The drawing under review shows one solid part. Ordinate dimensions are in mm from its lowest x, y, z. A direction names the side the tool comes from. Round coordinates to 2 decimals unless told otherwise and drop trailing zeros. Loops run counter-clockwise (first coordinate to the right, second up) from the corner with the lowest first, then second, coordinate; pieces in that order, holes last. Notation, with made-up numbers: M 37.25,6.25 L 46.25,6.25 A29 cw 46.25,34.25 Z; hole C 55.25,-30.5 d9. An arc over 180 degrees is marked long. Use a Markdown table: item, result.
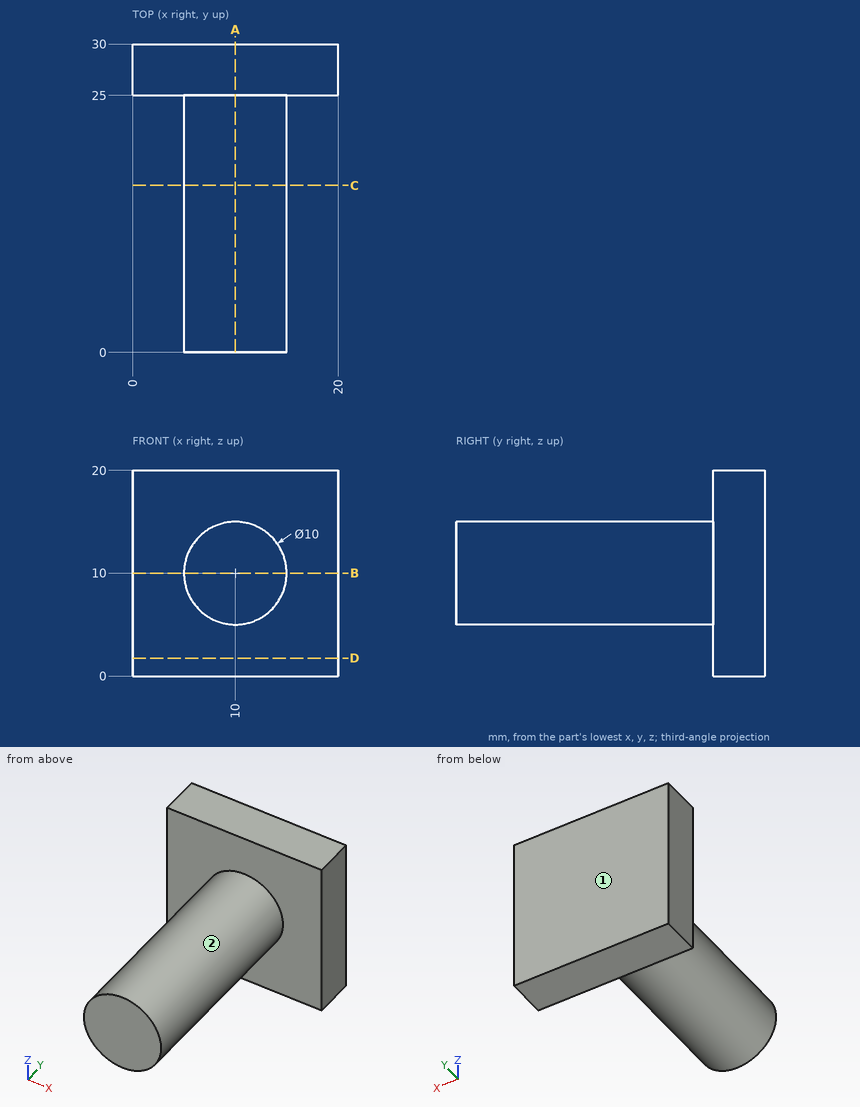
1. Take a section at D-D on z = 1.75. Give the boundary of the cut face in (x, y).
Check values:
| item | result |
|---|---|
| outline | M 0,25 L 20,25 L 20,30 L 0,30 Z |
2. Take a section at B-B on z = 10. Give the boundary of the cut face in (x, y), and give its area (3 significant figures).
Check values:
| item | result |
|---|---|
| outline | M 0,25 L 5,25 L 5,0 L 15,0 L 15,25 L 20,25 L 20,30 L 0,30 Z |
| area | 350 mm² |
3. Wall thickness on line 1 along Y through (x, z) = (15.5, 4.5); line 2 along Z through (x, y) = (7.5, 20); line 3 along X through (y, z) = (7.5, 9.25): over which ranges is each line inside the solid? List them lowest first. Write a range as from..to.
Check values:
| item | result |
|---|---|
| line 1 | y = 25..30 |
| line 2 | z = 5.67..14.33 |
| line 3 | x = 5.06..14.94 |
4. Take a section at A-A on x = 10. Give the boundary of the cut face in (y, z), and give its area (3 significant figures).
Check values:
| item | result |
|---|---|
| outline | M 0,5 L 25,5 L 25,0 L 30,0 L 30,20 L 25,20 L 25,15 L 0,15 Z |
| area | 350 mm² |
5. Take a section at C-C on y = 16.25. Give the boundary of the cut face in (x, z), and give its area (3 significant figures).
Check values:
| item | result |
|---|---|
| outline | C 10,10 d10 |
| area | 78.5 mm² |
6. Machinability: for the marked faces 1 and 2, which of the approach directions +Z, -Z, +X, -X, +Y, -Y give a long, thin tool a straight path to every point of the face, cutting with its end or side? Answer none if there is none.
Check values:
| item | result |
|---|---|
| face 1 | +Z, -Z, +X, -X, +Y |
| face 2 | -Y |
7. Insertion check: pin 1 (8 mm diameter, centred on x = 4.5, y = 3.5, fed in from -Z); pin 2 (12 mm diameter, centred on y = 13, z = 5.5, fed in from +X); pin 3 (6 mm diameter, centred on x = 14, y = 7.5, fed in from +Z). Each pin has a flat end and moves straight along its axis. Give the tip position at first contact, or say it passes through.
Check values:
| item | result |
|---|---|
| pin 1 | stops at z = 5.23 |
| pin 2 | stops at x = 15 |
| pin 3 | stops at z = 14.9 |
